CAD build for the part. Positions are in the model's coordinates, mm. Face numbers are marked on the shaded views. A direction names the side the tool comes from. Coordinates: 2 decimals unless noted, no trailing zeros. Order: outer loops, then holes, each group sorted by start corner. A loop starts at its lowest first (then second) coordinate and runs counter-clockwise, first axis right, second up. Notation, with made-up numbers: M 8,44.25 L 60,44.25 A25 cw 60,77.25 Z; hole C 0.5,-32.5 d8. An arc over 180 degrees is marked long. Write item = value, one per line.
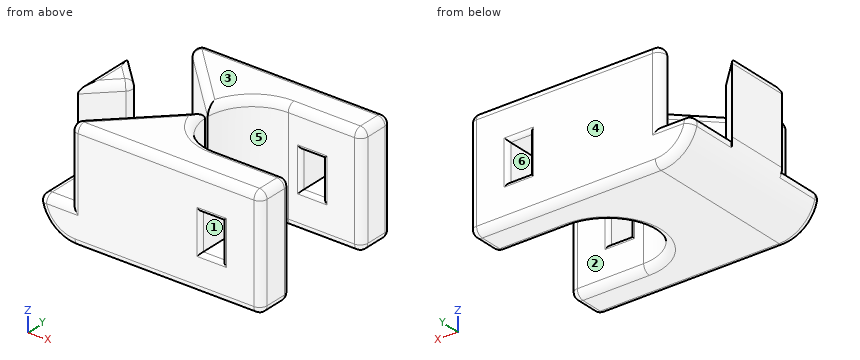
from build123d import *

# Parameters (mm, degrees)
PAD_DEPTH       = 15
POCKET_DEPTH    = 10
FILLET_R        = 5
SKETCH002_W     = 3
SKETCH002_H     = 5
POCKET001_DEPTH = 22.501
FILLET001_R     = 1
FILLET002_R     = 0.5


with BuildPart() as part:
    # Sketch → Pad (new body)
    with BuildSketch(Plane.XY):
        with BuildLine():
            ThreePointArc((20.25, 17.5), (14, 11.25), (20.25, 5))
            Line((30.25, 5), (20.25, 5))
            Line((30.25, 0), (30.25, 5))
            Line((0, 0), (30.25, 0))
            Line((0, 22.5), (0, 0))
            Line((30.25, 22.5), (0, 22.5))
            Line((30.25, 17.5), (30.25, 22.5))
            Line((20.25, 17.5), (30.25, 17.5))
        make_face()
    extrude(amount=PAD_DEPTH)

    # Sketch001 (on Face10 of Pad) → Pocket (cut)
    with BuildSketch(Plane.XY.offset(15)):
        Polygon((-0.75, 16.35), (-0.75, 26.25), (14.25, 11.25), (-0.75, -3.75), (-0.75, 6.15), (4.35, 11.25), align=None)
    extrude(amount=-POCKET_DEPTH, mode=Mode.SUBTRACT)

    # Fillet
    fillet_edges = [part.edges().sort_by_distance(p)[0] for p in [
        (0, 11.25, 0),
    ]]
    fillet(fillet_edges, radius=FILLET_R)

    # Sketch002 (on Face2 of Fillet) → Pocket001 (cut, through all)
    with BuildSketch(Plane.XZ):
        with Locations((23.5, 7.5)):
            Rectangle(SKETCH002_W, SKETCH002_H)
    extrude(amount=-POCKET001_DEPTH, mode=Mode.SUBTRACT)

    # Fillet001
    fillet001_edges = [part.edges().sort_by_distance(p)[0] for p in [
        (17.625, 22.5, 0),
        (30.25, 22.5, 7.5),
        (30.25, 17.5, 7.5),
        (30.25, 20, 0),
        (30.25, 20, 15),
        (25.25, 17.5, 0),
        (14, 11.25, 0),
        (25.25, 5, 0),
        (30.25, 5, 7.5),
        (30.25, 2.5, 0),
        (30.25, 0, 7.5),
        (30.25, 2.5, 15),
        (17.625, 0, 0),
        (16.625, 0, 15),
        (16.625, 22.5, 15),
        (15.918137, 6.744729, 15),
        (15.918137, 15.755271, 15),
        (25.25, 17.5, 15),
        (25.25, 5, 15),
        (8.502406, 16.997594, 15),
        (8.502406, 5.502406, 15),
        (4.35, 11.25, 10),
        (2.175, 13.425, 15),
        (0, 11.25, 15),
        (3, 22.5, 10),
        (3, 0, 10),
        (0, 3.45, 5),
        (1.5, 0, 5),
        (2.175, 9.075, 15),
        (1.5, 22.5, 5),
        (0, 19.05, 5),
    ]]
    fillet(fillet001_edges, radius=FILLET001_R)

    # Fillet002
    fillet002_edges = [part.edges().sort_by_distance(p)[0] for p in [
        (23.5, 22.5, 10),
        (22, 22.5, 7.5),
        (23.5, 22.5, 5),
        (25, 22.5, 7.5),
        (25, 5, 7.5),
        (23.5, 5, 10),
        (22, 5, 7.5),
        (23.5, 5, 5),
        (23.5, 17.5, 10),
        (22, 17.5, 7.5),
        (23.5, 17.5, 5),
        (25, 17.5, 7.5),
        (23.5, 0, 10),
        (22, 0, 7.5),
        (23.5, 0, 5),
        (25, 0, 7.5),
    ]]
    fillet(fillet002_edges, radius=FILLET002_R)


solid = part.part
(1) Pull direction Y, two halves, no side cores. Call the marked faces 4, 5 and 6: +Y half, -Y half, draft (parallel to the pull), parting line (faces both ways), or undercut.
Evaluation:
face_4 = +Y half
face_5 = undercut
face_6 = draft
(2) Tool access for the marked faces 1, 2 and 3: list every direction of +Z, -Z, +X, -X, +Y, -Y with a clear straight run to the whole face (end or side of a thin tool).
Evaluation:
face_1 = +Y, -Y
face_2 = +Z, -Z, +X
face_3 = +Z, +X, -X, +Y, -Y
(3) Slice it at B-B, the plane z = 12.25. Write the cut outline in (x, y), then the cut area to 3 significant figures.
Evaluation:
outline = M 0,6.9 L 3.64,10.54 A1 ccw 3.64,11.96 L 0,15.6 Z; M 4.71,1.71 A1 ccw 5.41,0 L 29.25,0 A1 ccw 30.25,1 L 30.25,4 A1 ccw 29.25,5 L 20.25,5 A6.25 cw 14,11 Z; M 4.71,20.79 L 14,11.5 A6.25 cw 20.25,17.5 L 29.25,17.5 A1 ccw 30.25,18.5 L 30.25,21.5 A1 ccw 29.25,22.5 L 5.41,22.5 A1 ccw Z
area = 316 mm²
(4) Wall check: line 1 (Z direction, x = 23, y = 2.75); line 2 (Y direction, x = 28, z = 11); line 3 (Z direction, x = 6, y = 9.25). Give the ranges that are in metal, low to high. Write a range as from..to.
Evaluation:
line_1 = 0..5, 10..15
line_2 = 0..5, 17.5..22.5
line_3 = 0..5
(5) Pin check, flat tips, straight feed: pin 1 Ø2 at (y, z) = (3.5, 6.5) entering from -X; pin 2 Ø1.2 at (y, z) = (20, 7) entering from -X; pin 3 Ø1.5 at (x, y) = (3, 15.5) entering from -Z. Stop position of each tip, or through.
Evaluation:
pin_1 = 5.5
pin_2 = 4.9
pin_3 = 0.16
(6) Slice it at C-C, the plane x = 23. State how many separate pieces and enclosed holes the cut face has, then the cut area to 3 significant figures.
Evaluation:
separate_pieces = 4
enclosed_holes = 0
area = 97.9 mm²
(7) Slice it at A-A, the plane x = 27.5. Write the cut outline in (y, z).
Evaluation:
outline = M 0,1 A1 ccw 1,0 L 4,0 A1 ccw 5,1 L 5,14 A1 ccw 4,15 L 1,15 A1 ccw 0,14 Z; M 17.5,1 A1 ccw 18.5,0 L 21.5,0 A1 ccw 22.5,1 L 22.5,14 A1 ccw 21.5,15 L 18.5,15 A1 ccw 17.5,14 Z
